Model file for the job. Use its own axes, mm. A direction names the side the tool comes from. Coordinates: 2 decimals unless noted, no trailing zeros. Order: outer loops, then holes, each group sorted by start corner. A loop starts at its lowest first (then second) coordinate and runs counter-clockwise, first axis right, second up. Notation, with made-up numbers: (-14, 45.5) -> (41, 45.5) arc R22 ccw to (41, 64.5) -> close; hole circle Ø1 at (3, 69). An arc over 180 degrees is marked (long way). Use CSV: the item, a comma, the result in double quotes. Start each with the question number.
(1) Cut at B-B on y = 67. Write the cut outline in (x, z), plus the area to 3 significant figures.
(2) Probe L1, parallel to X at y = 67, z = -13; L2, parallel to Y at x = 295, z = -3.6; L3, parallel to X at y = 74.5, z = -4.75. List the from-to ranges inside material, lowest first.
(3) Pull direction X, two halves, no side cores. Call faces 1 (the cylindrical face through (77.6, 65.2, -12.1)), 2 (the flat face through (185, 52, -18)), 3 (the flat face through (345, 50, -9)): pulls with the +X half, pulls with the -X half, needs draft (parallel to the pull), parting line crosses it, or undercut.
(4) Cut at A-A on x = 80. Write the cut outline in (y, z), plus the area to 3 significant figures.
(5) Tool access for faces 4 (the flat face through (185, 92, -9)), 5 (the cylindrical face through (89.061, 69.854, -2.958)): list every direction of +Z, -Z, +X, -X, +Y, -Y with a clear straight run to the whole face (end or side of a thin tool).
(6) Pin check, flat tips, straight feed: pin 1 Ø5 at (x, y) = (80, 67) entering from -Z; pin 2 Ø9.5 at (x, y) = (295, 67) entering from +Z. Stop position of each tip, or through.
```python
from build123d import *

# Parameters (mm, degrees)
SKETCH002_W  = 315
SKETCH002_H  = 82
SKETCH002_R  = 3
PAD002_DEPTH = 18
SKETCH003_R  = 9.5
POCKET_DEPTH = 6


with BuildPart() as part:
    # Sketch002 → Pad002 (new body)
    with BuildSketch(Plane.XY):
        with Locations((0, 41)):
            Rectangle(SKETCH002_W, SKETCH002_H)
        with Locations((-107.5, 57)):
            Circle(SKETCH002_R, mode=Mode.SUBTRACT)
        with Locations((107.5, 57)):
            Circle(SKETCH002_R, mode=Mode.SUBTRACT)
    extrude(amount=PAD002_DEPTH)

    # Sketch003 (on Face8 of Pad002) → Pocket (cut)
    with BuildSketch(Plane.XY.offset(18)):
        with Locations((-107.5, 57)):
            Circle(SKETCH003_R)
    pocket = extrude(amount=-POCKET_DEPTH, mode=Mode.SUBTRACT)

    # Mirrored: Pocket across Sketch003 V_Axis
    add(pocket.mirror(Plane(origin=(0, 0, 18), x_dir=(0, 0, 1), z_dir=(1, 0, 0))), mode=Mode.SUBTRACT)


with BuildPart() as part_1:
    # Clone placement: moved
    add(part.part.moved(Location((187.5, 10, -18))))


solid = part_1.part
```
Outcome:
1,outline,"(30, -18) -> (77, -18) -> (77, -6) -> (70.5, -6) -> (70.5, 0) -> (30, 0) -> close; (83, -18) -> (292, -18) -> (292, -6) -> (285.5, -6) -> (285.5, 0) -> (89.5, 0) -> (89.5, -6) -> (83, -6) -> close; (298, -18) -> (345, -18) -> (345, 0) -> (304.5, 0) -> (304.5, -6) -> (298, -6) -> close"
1,area,"5,300 mm2"
2,L1,"30 to 77, 83 to 292, 298 to 345"
2,L2,"10 to 57.5, 76.5 to 92"
2,L3,"30 to 74.17, 85.83 to 289.17, 300.83 to 345"
3,face 1,"undercut"
3,face 2,"needs draft"
3,face 3,"pulls with the +X half"
4,outline,"(10, -18) -> (64, -18) -> (64, -6) -> (57.5, -6) -> (57.5, 0) -> (10, 0) -> close; (70, -18) -> (92, -18) -> (92, 0) -> (76.5, 0) -> (76.5, -6) -> (70, -6) -> close"
4,area,"1,290 mm2"
5,face 4,"+Z, -Z, +X, -X, +Y"
5,face 5,"+Z"
6,pin 1,"through"
6,pin 2,"z = -6"
